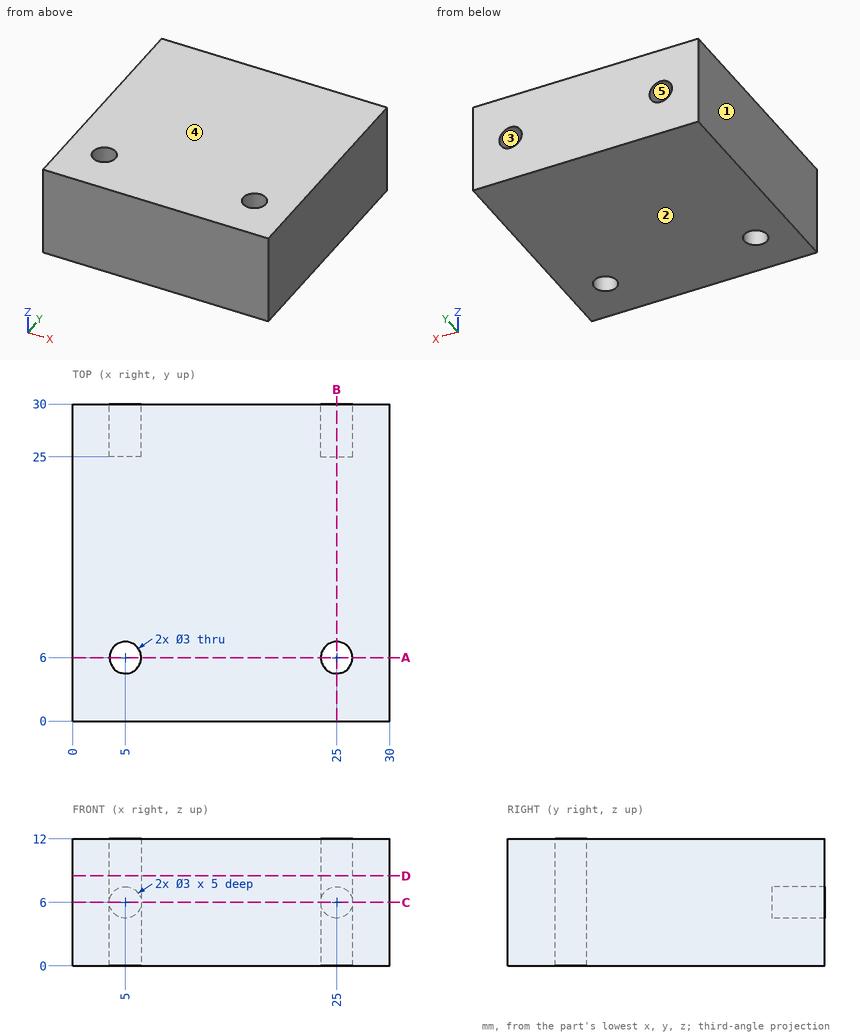
Could you check a few things on this drawing? It's one solid part, dimensions in mm from its lowest x, y, z. A direction names the side the tool comes from. Coordinates: 2 decimals unless noted, no trailing zeros. Order: outer loops, then holes, each group sorted by start corner. A loop starts at its lowest first (then second) coordinate and runs counter-clockwise, first axis right, second up. Notation, with made-up numbers: (72.5, 17) -> (97.5, 17) arc R23 ccw to (97.5, 29) -> close; hole circle Ø4 at (54, -3.75). An arc over 180 degrees is marked (long way). One line per item, written item: value. Start each with the question number.
1) Imagine slicing it at D-D on z = 8.5. List the corners of the cut face in (x, y) for me.
2) Which directions (+Z, -Z, +X, -X, +Y, -Y) give clear straight access to the entire face, cutting with the end or side of a thin tool? Please do the marked faces 4 and 5.
3) Imagine slicing it at C-C on z = 6. List the corners of the cut face in (x, y) for me.
4) Imagine slicing it at B-B on x = 25. List the corners of the cut face in (y, z) for me, plus the area to 3 significant figures.
5) We'd pull the mould along X, two halves only. Please class the marked faces 1, 2 and 3: +X half, -X half, draft (parallel to the pull), parting line (faces both ways), or undercut.
6) I'm going to push flat-ended pins straight in: pin 1 (2.5 mm diameter, centred on x = 5, y = 6, fed in from +Z); pin 2 (0.9 mm diameter, centred on x = 24.5, z = 5.5, fed in from +Y). Where does each tip first touch, or does it pass through?
7) If I drill on L1, parallel to X at y = 27.2, z = 6; L2, parallel to Z at x = 25, y = 26.6; L3, parallel to Y at x = 5, z = 9.25, over which ranges is the centre line in solid material (lowest first)? Write a range as [from, to].
8) Imagine slicing it at A-A on y = 6. List the corners of the cut face in (x, z) for me.
Answer list:
1. outline: (0, 0) -> (30, 0) -> (30, 30) -> (0, 30) -> close; hole circle Ø3 at (5, 6); hole circle Ø3 at (25, 6)
2. face 4: +Z, +X, -X, +Y, -Y
2. face 5: +Y
3. outline: (0, 0) -> (30, 0) -> (30, 30) -> (26.5, 30) -> (26.5, 25) -> (23.5, 25) -> (23.5, 30) -> (6.5, 30) -> (6.5, 25) -> (3.5, 25) -> (3.5, 30) -> (0, 30) -> close; hole circle Ø3 at (5, 6); hole circle Ø3 at (25, 6)
4. outline: (0, 0) -> (4.5, 0) -> (4.5, 12) -> (0, 12) -> close; (7.5, 0) -> (30, 0) -> (30, 4.5) -> (25, 4.5) -> (25, 7.5) -> (30, 7.5) -> (30, 12) -> (7.5, 12) -> close
4. area: 309 mm2
5. face 1: -X half
5. face 2: draft
5. face 3: undercut
6. pin 1: passes through
6. pin 2: stops at y = 25
7. L1: x = [0, 3.5], [6.5, 23.5], [26.5, 30]
7. L2: z = [0, 4.5], [7.5, 12]
7. L3: y = [0, 4.5], [7.5, 30]
8. outline: (0, 0) -> (3.5, 0) -> (3.5, 12) -> (0, 12) -> close; (6.5, 0) -> (23.5, 0) -> (23.5, 12) -> (6.5, 12) -> close; (26.5, 0) -> (30, 0) -> (30, 12) -> (26.5, 12) -> close
